For this review, use the dimensioned drawing (mm, ordinates from the lowest corner) and the shaded views. A direction names the side the tool comes from. Coordinates: 2 decimals unless noted, no trailing zeros. Write each loop counter-clockwise with the first axis right and the second up, starting at its lowest first coordinate (ties: lowest second). Pieces come first, ordered by that corner, then holes. Notation, with made-up numbers: (59.5, -24.75) - (77.5, -24.75) arc R26 cw to (77.5, 13.25) - close; hole circle Ø8 at (22.5, 60.5). An arc over 180 degrees is marked (long way). One line per item, written item: value.
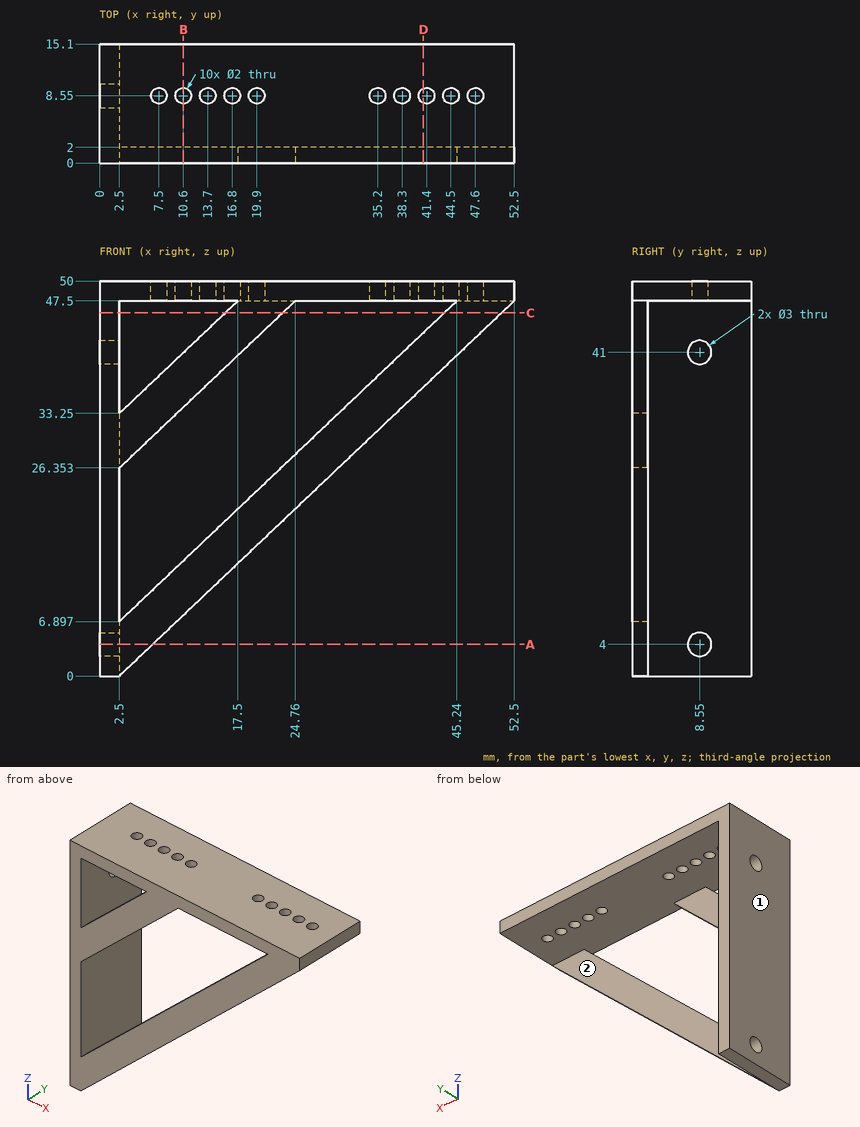
1. Consider section D-D, the plane x = 41. Write out the cut boundary in (y, z) (1 decimal).
Answer block:
outline: (0, 36.6) - (2, 36.6) - (2, 43.5) - (0, 43.5) - close; (0, 47.5) - (7.6, 47.5) - (7.6, 50) - (0, 50) - close; (9.5, 47.5) - (15.1, 47.5) - (15.1, 50) - (9.5, 50) - close
2. For the marked faces 1 and 2, list the 3-axis set-ups (+Z, -Z, +X, -X, +Y, -Y) from which the entire face can be reached by the end or side of a thin tool; tool diameter is ignored.
Answer block:
face 1: +Z, -Z, -X, +Y, -Y
face 2: -Z, +X, +Y
3. Consider section A-A, the plane z = 4. Write out the cut boundary in (x, y).
Answer block:
outline: (0, 0) - (6.71, 0) - (6.71, 2) - (2.5, 2) - (2.5, 7.05) - (0, 7.05) - close; (0, 10.05) - (2.5, 10.05) - (2.5, 15.1) - (0, 15.1) - close
4. Consider section C-C, the plane z = 46. Write out the cut boundary in (x, y).
Answer block:
outline: (0, 0) - (2.5, 0) - (2.5, 15.1) - (0, 15.1) - close; (15.92, 0) - (23.18, 0) - (23.18, 2) - (15.92, 2) - close; (43.66, 0) - (50.92, 0) - (50.92, 2) - (43.66, 2) - close
5. Consider section B-B, the plane x = 10.6. Give the number of separate pieces and of enclosed holes in the cut face.
Answer block:
separate pieces: 4
enclosed holes: 0
6. Insertion check: pin 1 Ø4 at (y, z) = (8.55, 4) entering from +X; pin 2 Ø2.5 at (x, y) = (38.3, 8.55) entering from +Z; pin 3 Ø6 at (x, y) = (24, 3.5) entering from -Z (1 decimal); pin 4 Ø3 at (x, y) = (10.5, 6.5) entering from -Z. Each pin has a flat end and moves straight along its axis. Give the tip position at first contact, or say it passes through.
Answer block:
pin 1: stops at x = 2.5
pin 2: stops at z = 50
pin 3: stops at z = 18
pin 4: stops at z = 47.5
7. Wall thickness on line 1 along Y through (x, z) = (7.5, 49.1); line 2 along Y through (x, z) = (1.8, 41); line 3 along Z through (x, y) = (18, 5.5): over which ranges is each line inside the solid? List them lowest first.
Answer block:
line 1: y = 0 to 7.55, 9.55 to 15.1
line 2: y = 0 to 7.05, 10.05 to 15.1
line 3: z = 47.5 to 50
